```python
from build123d import *

# Parameters (mm, degrees)
SKETCH2_R           = 2.612661588
BOSS_EXTRUDE1_DEPTH = 2
CHAMFER1_SIZE       = 0.25


with BuildPart() as part:
    # Sketch1 → Revolve1 (revolve)
    with BuildSketch(Plane.XY):
        Polygon((0.2, -3.5), (0.2, -2.9), (0.75, -1.947372056), (0.75, 3), (1.100103769, 3.5), (2.25, 3.5), (2.25, 2.5), (2.5, 2.5), (2.5, 0.25), (2.25, 0.25), (2.25, -0.5), (3, -0.5), (3, -2.5), (1.100207538, -2.5), (0.4, -3.5), align=None)
    revolve(axis=Axis((0, -3.5, 0), (0, 1, 0)))

    # Sketch2 → Boss-Extrude1 (add)
    with BuildSketch(Plane.XZ.offset(2.5)):
        Polygon((1.732050808, 3), (-1.732050808, 3), (-3.464101615, 0), (-1.732050808, -3), (1.732050808, -3), (3.464101615, 0), align=None)
        Circle(SKETCH2_R, mode=Mode.SUBTRACT)
    extrude(amount=-BOSS_EXTRUDE1_DEPTH)

    # Chamfer1
    chamfer1_edges = [part.edges().sort_by_distance(p)[0] for p in [
        (-2.25, 3.5, 0),
    ]]
    chamfer(chamfer1_edges, length=CHAMFER1_SIZE)


solid = part.part
```
Input: part model. Units: mm. Frame: model coordinates. A direction names the side the tool comes from. Coordinates: 2 decimals unless noted, no trailing zeros. Loops run counter-clockwise (first coordinate to the right, second up) from the corner with the lowest first, then second, coordinate; pieces in that order, holes last. Notation, with made-up numbers: (47.25, 84) -> (72.25, 84) arc R9 ccw to (72.25, 100) -> close; hole circle Ø6 at (-17, 18). An arc over 180 degrees is marked (long way). Use a Markdown table: item, result.
1) Access query for faces 1 (the cylindrical face through (-0.29, -0.13, -2.23)), 2 (the cylindrical face through (-0.54, 1.36, 2.44)), 3 (the flat face through (1.5, -2.5, 0)). Directions: +Z, -Z, +X, -X, +Y, -Y. A direction counts if a zero-diameter tool reaches every point of the face in a straight line with its end or side. Return the directions, or none.
Results found:
| item | result |
|---|---|
| face 1 | none |
| face 2 | +Y |
| face 3 | -Y |
2) Contact query for flat-ended pins moving along their axis: pin 1 (0.9 mm diameter, centred on x = 0, z = 0, fed in from +Y); pin 2 (2 mm diameter, centred on x = -2.5, y = 2.5, fed in from -Z); pin 3 (1 mm diameter, centred on x = 1, z = 1, fed in from -Y). Output: stop coordinate, or through.
Results found:
| item | result |
|---|---|
| pin 1 | stops at y = -2.47 |
| pin 2 | stops at z = -2 |
| pin 3 | stops at y = -2.77 |
3) Cut plane D-D (y = 2.75). Return the cut outline in (x, z), then the cut area to 3 significant figures.
Results found:
| item | result |
|---|---|
| outline | circle Ø4.5 at (0, 0); hole circle Ø1.5 at (0, 0) |
| area | 14.1 mm2 |
4) Pull-direction query (X, two-part tool) for faces 4 (the flat face through (2.6, -1.5, -1.5)), 5 (the flat face through (0, -2, -3)), 6 (the conical face through (0.34, -2.63, -0.11)); classes: released by +X, released by -X, zero draft, split by the parting line, or undercut.
Results found:
| item | result |
|---|---|
| face 4 | released by +X |
| face 5 | zero draft |
| face 6 | undercut |
5) Cut plane C-C (y = 1.25). Return the cut outline in (x, z), then the cut area to 3 significant figures.
Results found:
| item | result |
|---|---|
| outline | circle Ø5 at (0, 0); hole circle Ø1.5 at (0, 0) |
| area | 17.9 mm2 |
6) Material intervals for line 1 along X through (y, z) = (0.75, 0); line 2 along Y through (x, z) = (1.5, -1.8), sorted ascending. Write a range as from..to.
Results found:
| item | result |
|---|---|
| line 1 | x = -2.5..-0.75, 0.75..2.5 |
| line 2 | y = -2.5..-0.5, 0.25..2.5 |
7) Cut plane B-B (z = 2.35). Return the cut outline in (x, y), then the cut area to 3 significant figures.
Results found:
| item | result |
|---|---|
| outline | (-2.11, -2.5) -> (2.11, -2.5) -> (2.11, -0.5) -> (-2.11, -0.5) -> close; (-0.85, 0.25) -> (0.85, 0.25) -> (0.85, 2.5) -> (-0.85, 2.5) -> close |
| area | 12.3 mm2 |
